Could you check a few things on this model? Use its own coordinates, in mm. Face numbers are marked on the shaded views. A direction names the side the tool comes from. Coordinates: 2 decimals unless noted, no trailing zeros. Write each loop counter-clockwise with the first axis right and the second up, starting at its lowest first coordinate (ties: lowest second). Pieces come first, ordered by that corner, then holes.
```python
from build123d import *

# Parameters (mm, degrees)
F3_W        = 29.1
F3_H        = 38.6
F4_DEPTH    = 6
F5_T        = 2
F7_DEPTH    = 0.5
F8_T1_DEPTH = 4.571682988
F8_T3_DEPTH = 4.571682988
F9_W        = 10.1
F9_H        = 9.4
F10_DEPTH   = 4


# Not quite as in the source:
# - a fillet or chamfer that OpenCascade refuses, or shapes differently, is made with other operations: its cross-section is extruded or revolved along the edge and cut away or added
# - a feature of the source that left no trace in its solid (it failed there, or was rolled back) is left out
# - a shell that OpenCascade refuses in one call is made with other operations: the cavity is built on its own and cut out


with BuildPart() as f4:
    # F3 (on Front) → F4 (new body)
    with BuildSketch(Plane.XZ):
        Rectangle(F3_W, F3_H)
        with BuildLine():
            Line((-12.55, -17.3), (-12.55, -6.7))
            Line((-12.55, -6.7), (-9.85, -6.7))
            Line((-9.85, -6.7), (-9.85, -8.6))
            ThreePointArc((-9.85, -8.6), (-9.3575419845, -9.4628939105), (-9.65, -10.4124038405))
            Line((-9.65, -10.4124038405), (-9.05, -11.8))
            Line((-9.05, -11.8), (-7.05, -11.8))
            Line((-7.05, -11.8), (-7.05, -17.3))
            Line((-7.05, -17.3), (-12.55, -17.3))
        make_face(mode=Mode.SUBTRACT)
        with BuildLine():
            Line((12.55, -6.7), (12.55, -17.3))
            Line((12.55, -17.3), (7.05, -17.3))
            Line((7.05, -17.3), (7.05, -11.8))
            Line((7.05, -11.8), (9.05, -11.8))
            Line((9.05, -11.8), (9.65, -10.4124038405))
            ThreePointArc((9.65, -10.4124038405), (9.3575419845, -9.4628939105), (9.85, -8.6))
            Line((9.85, -8.6), (9.85, -6.7))
            Line((9.85, -6.7), (12.55, -6.7))
        make_face(mode=Mode.SUBTRACT)
        with BuildLine():
            Line((-12.55, 6.7), (-12.55, 17.3))
            Line((-12.55, 17.3), (-9.85, 17.3))
            Line((-9.85, 17.3), (-9.85, 15.4))
            ThreePointArc((-9.85, 15.4), (-9.3575419845, 14.5371060895), (-9.65, 13.5875961595))
            Line((-9.65, 13.5875961595), (-9.05, 12.2))
            Line((-9.05, 12.2), (-7.05, 12.2))
            Line((-7.05, 12.2), (-7.05, 6.7))
            Line((-7.05, 6.7), (-12.55, 6.7))
        make_face(mode=Mode.SUBTRACT)
        with BuildLine():
            Line((7.05, 6.7), (7.05, 12.2))
            Line((7.05, 12.2), (9.05, 12.2))
            Line((9.05, 12.2), (9.65, 13.5875961595))
            ThreePointArc((9.65, 13.5875961595), (9.3575419845, 14.5371060895), (9.85, 15.4))
            Line((9.85, 15.4), (9.85, 17.3))
            Line((9.85, 17.3), (12.55, 17.3))
            Line((12.55, 17.3), (12.55, 6.7))
            Line((12.55, 6.7), (7.05, 6.7))
        make_face(mode=Mode.SUBTRACT)
    extrude(amount=F4_DEPTH)

    # F5: shell of thickness 2, made by hand


with BuildPart() as f5_core1:
    # F5_t2: copy of F4
    add(f4.part)

    # the walls: a layer under each face that stays
    f5_faces = [f5_core1.faces().sort_by_distance(p)[0] for p in [
        (14.55, -3, 0),
        (0, -3, 19.3),
        (-14.55, -3, 0),
        (0, -3, -19.3),
        (0, -6, 0),
    ]]
    thicken(f5_faces, amount=-F5_T, mode=Mode.SUBTRACT)


with BuildPart() as f4_1:
    add(f4.part)

    # what is left inside the walls is the cavity
    f5_cavity = [f5_core1.part.solids().sort_by_distance(p)[0] for p in [
        (0, -0.02, -5.766667),
    ]]
    add(f5_cavity, mode=Mode.SUBTRACT)

    # F6 (on face) → F7 (join)
    with BuildSketch(Plane(origin=(0, -4, 0), x_dir=(-1, 0, 0), z_dir=(0, 1, 0))):
        with BuildLine():
            Line((-7.05, 17.3), (-9.85, 17.3))
            Line((-9.85, 17.3), (-9.85, 15.4))
            ThreePointArc((-9.85, 15.4), (-9.3575419845, 14.5371060895), (-9.65, 13.5875961595))
            Line((-9.65, 13.5875961595), (-9.05, 12.2))
            Line((-9.05, 12.2), (-7.05, 12.2))
            Line((-7.05, 12.2), (-7.05, 17.3))
        make_face()
        with BuildLine():
            Line((9.85, 17.3), (7.05, 17.3))
            Line((7.05, 17.3), (7.05, 12.2))
            Line((7.05, 12.2), (9.05, 12.2))
            Line((9.05, 12.2), (9.65, 13.5875961595))
            ThreePointArc((9.65, 13.5875961595), (9.3575419845, 14.5371060895), (9.85, 15.4))
            Line((9.85, 15.4), (9.85, 17.3))
        make_face()
        with BuildLine():
            Line((-9.65, -10.4124038405), (-9.05, -11.8))
            Line((-9.05, -11.8), (-7.05, -11.8))
            Line((-7.05, -11.8), (-7.05, -6.7))
            Line((-7.05, -6.7), (-9.85, -6.7))
            Line((-9.85, -6.7), (-9.85, -8.6))
            ThreePointArc((-9.85, -8.6), (-9.3575419845, -9.4628939105), (-9.65, -10.4124038405))
        make_face()
        with BuildLine():
            Line((9.85, -6.7), (7.05, -6.7))
            Line((7.05, -6.7), (7.05, -11.8))
            Line((7.05, -11.8), (9.05, -11.8))
            Line((9.05, -11.8), (9.65, -10.4124038405))
            ThreePointArc((9.65, -10.4124038405), (9.3575419845, -9.4628939105), (9.85, -8.6))
            Line((9.85, -8.6), (9.85, -6.7))
        make_face()
    extrude(amount=F7_DEPTH)

    # F8: chamfer of 1 on 4 edges, made by hand

    # F8_s2 → F8_t1 (cut)
    with BuildSketch(Plane.YZ.offset(7.05)):
        Polygon((-3.5, -10.8), (-4.5, -11.8), (-3.5, -11.8), align=None)
        Polygon((-3.5, 13.2), (-4.5, 12.2), (-3.5, 12.2), align=None)
    extrude(amount=F8_T1_DEPTH, mode=Mode.SUBTRACT)

    # F8_s4 → F8_t3 (cut)
    with BuildSketch(Plane.YZ.offset(-11.621682988)):
        Polygon((-3.5, -10.8), (-4.5, -11.8), (-3.5, -11.8), align=None)
        Polygon((-3.5, 13.2), (-4.5, 12.2), (-3.5, 12.2), align=None)
    extrude(amount=F8_T3_DEPTH, mode=Mode.SUBTRACT)

    # F9 (on face) → F10 (join, through all)
    with BuildSketch(Plane(origin=(0, -4, 0), x_dir=(-1, 0, 0), z_dir=(0, 1, 0))):
        Polygon((7.05, -17.3), (7.05, -11.3), (7.05, -6.7), (9.85, -6.7), (12.55, -6.7), (12.55, -4.7), (7.05, -4.7), (7.05, 4.7), (12.55, 4.7), (12.55, 6.7), (7.05, 6.7), (7.05, 12.7), (7.05, 17.3), (5.05, 17.3), (5.05, 6.7), (-5.05, 6.7), (-5.05, 17.3), (-7.05, 17.3), (-7.05, 12.7), (-7.05, 6.7), (-12.55, 6.7), (-12.55, 4.7), (-7.05, 4.7), (-7.05, -4.7), (-12.55, -4.7), (-12.55, -6.7), (-9.85, -6.7), (-7.05, -6.7), (-7.05, -11.3), (-7.05, -17.3), (-5.05, -17.3), (-5.05, -6.7), (5.05, -6.7), (5.05, -17.3), align=None)
        Rectangle(F9_W, F9_H, mode=Mode.SUBTRACT)
    extrude(amount=F10_DEPTH)


solid = f4_1.part
```
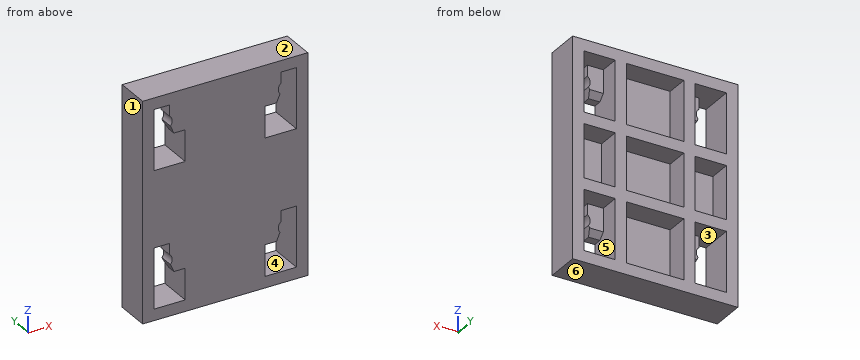
1. I want a section at B-B on z = 16. Please give me the cut outline in (x, y).
Verdict:
outline: (-14.55, -6) - (-12.55, -6) - (-12.55, 0) - (-14.55, 0) - close; (-9.85, -6) - (9.85, -6) - (9.85, -3.5) - (7.05, -3.5) - (7.05, 0) - (5.05, 0) - (5.05, -4) - (-5.05, -4) - (-5.05, 0) - (-7.05, 0) - (-7.05, -3.5) - (-9.85, -3.5) - close; (12.55, -6) - (14.55, -6) - (14.55, 0) - (12.55, 0) - close
2. I want a section at A-A on x = -11.25. Please give me the cut outline in (y, z).
Verdict:
outline: (-6, -19.3) - (0, -19.3) - (0, -17.3) - (-6, -17.3) - close; (-6, -6.7) - (0, -6.7) - (0, -4.7) - (-4, -4.7) - (-4, 4.7) - (0, 4.7) - (0, 6.7) - (-6, 6.7) - close; (-6, 17.3) - (0, 17.3) - (0, 19.3) - (-6, 19.3) - close
3. I want a section at C-C on x = 1.5. Please give me the cut outline in (y, z).
Verdict:
outline: (-6, -19.3) - (0, -19.3) - (0, -17.3) - (-4, -17.3) - (-4, -6.7) - (0, -6.7) - (0, -4.7) - (-4, -4.7) - (-4, 4.7) - (0, 4.7) - (0, 6.7) - (-4, 6.7) - (-4, 17.3) - (0, 17.3) - (0, 19.3) - (-6, 19.3) - close
4. On a 3-axis mill with a long thin cutter (end or side, diameter ignored), from which of +Z, -Z, +X, -X, +Y, -Y can I reach the whole of each face in a straight line? I mean the marked faces 4, 5 and 6. Say none if no direction works.
Verdict:
face 4: +Y, -Y
face 5: +Y
face 6: -Z, +X, -X, +Y, -Y
5. If we mould it in two halves opening along Z, with no side actions, what happens to the marked faces 1, 2 and 3? For each: pulls with the +Z half, pulls with the -Z half, needs draft (parallel to the pull), parting line crosses it, or undercut.
Verdict:
face 1: needs draft
face 2: pulls with the +Z half
face 3: undercut
6. I want a section at D-D on z = 4. Please give me the cut outline in (x, y), plus the area to 3 significant figures.
Verdict:
outline: (-14.55, -6) - (14.55, -6) - (14.55, 0) - (12.55, 0) - (12.55, -4) - (7.05, -4) - (7.05, 0) - (5.05, 0) - (5.05, -4) - (-5.05, -4) - (-5.05, 0) - (-7.05, 0) - (-7.05, -4) - (-12.55, -4) - (-12.55, 0) - (-14.55, 0) - close
area: 90.2 mm2
7. Please list where these lines run through material, in increasing order: line 1 along X through (y, z) = (-1.5, -15); line 2 along Z through (x, y) = (-9.5, -1.7); line 3 along X through (y, z) = (-4.5, -16).
Verdict:
line 1: x = -14.55 to -12.55, -7.05 to -5.05, 5.05 to 7.05, 12.55 to 14.55
line 2: z = -19.3 to -17.3, -6.7 to -4.7, 4.7 to 6.7, 17.3 to 19.3
line 3: x = -14.55 to -12.55, -7.05 to 7.05, 12.55 to 14.55
